Autodesk Inventor part; units mm, degrees
ref_plane "YZ Plane" through (0, 0, 0) normal (1, 0, 0) x (0, 1, 0)
ref_plane "XZ Plane" through (0, 0, 0) normal (0, 1, 0) x (-1, 0, 0)
ref_plane "XY Plane" through (0, 0, 0) normal (0, 0, 1) x (1, 0, 0)
sketch "スケッチ1" plane through (0, 0, 0) normal (0, 1, 0) x (-1, 0, 0)
  circle A0 centre (0, 0) radius 125
  dimension "d0" = 250
extrude "押し出し1" add sketch "スケッチ1" along normal blind 3
sketch "スケッチ2" plane through (0, 3, 0) normal (0, 1, 0) x (1, 0, 0)
  circle A0 centre (0, 0) radius 125
  circle A1 centre (0, 0) radius 117.5
  dimension "d3" = 250
  dimension "d4" = 235
extrude "押し出し2" add sketch "スケッチ2" along normal blind 144
sketch "スケッチ3" plane through (0, 147, 0) normal (0, 1, 0) x (1, 0, 0)
  circle A0 centre (0, 0) radius 125
extrude "押し出し3" add sketch "スケッチ3" along normal blind 3
sketch "スケッチ4" plane through (0, 150, 0) normal (0, 1, 0) x (1, 0, 0)
  circle A0 centre (60, 60) radius 15
  point P0 (0, 0)
  dimension "d9" = 30
  dimension "d10" = 60
  dimension "d11" = 60
extrude "押し出し4" cut sketch "スケッチ4" against normal through all
properties part number "dummy1"
Could you check a few things on this model? Use its own coordinates, in mm. A direction names the side the tool comes from. Round coordinates to 2 decimals unless told otherwise and drop trailing zeros. Order: outer loops, then holes, each group sorted by start corner. A loop starts at its lowest first (then second) coordinate and runs counter-clockwise, first axis right, second up. Notation, with made-up numbers: M 88,54.25 L 136,54.25 A11 cw 136,71.25 Z; hole C -38.75,34 d5. An arc over 180 degrees is marked long. One line per question, with ' | ' between items. Start each with the question number.
(1) For faces 1 (the face through (2, 3, 2)), 2 (the face through (-2, 150, -2)), which set-ups out of +Z, -Z, +X, -X, +Y, -Y let a thin tool reach every point of the face, with its end or its side?
(2) Suppose I cut it at B-B on y = 35.5. List the corners of the cut face in (x, z) for me, then the cut area to 3 significant figures.
(3) Please list where these lines run through material, in increasing order: line 1 along Y through (x, z) = (31.5, -79.5); line 2 along Z through (x, y) = (0, 70.5).
(4) Suppose I cut it at D-D on z = -12. List the corners of the cut face in (x, y) for me.
(5) Suppose I cut it at A-A on z = -38. List the corners of the cut face in (x, y) for me.
(6) Thinking about a two-plate mould opening in Z: for faces 3 (the face through (56.748, 1.521, -45.357)), 4 (the face through (-2, 147, -2)), 5 (the face through (2, 0, 2)), which applies, +Z half, -Z half, draft (parallel to the pull), parting line (faces both ways), or undercut?
(7) For P1, Ø5, axis at y = 130.5, z = 66.5, coming from the +X side; P2, Ø10, axis at y = 113, z = -94.5, coming from the -X side; P3, Ø1, axis at y = 16, z = -75, coming from the -X side; P4, Ø24, axis at x = 60, z = -60, coming from the -Y side, each with a flat end and sliding along its axis, tell me the tip position at first contact or that it passes through.
Geometry results:
1) face 1: none | face 2: +Z, -Z, +X, -X, +Y
2) outline: C 0,0 d250; hole C 0,0 d235 | area: 5,710 mm²
3) line 1: 0 to 3, 147 to 150 | line 2: -125 to -117.5, 117.5 to 125
4) outline: M -124.42,0 L 124.42,0 L 124.42,150 L -124.42,150 Z; hole M -116.89,3 L 116.89,3 L 116.89,147 L -116.89,147 Z
5) outline: M -119.08,0 L 119.08,0 L 119.08,150 L -119.08,150 Z; hole M -111.19,3 L 111.19,3 L 111.19,147 L -111.19,147 Z
6) face 3: undercut | face 4: undercut | face 5: draft
7) P1: x = 107.37 | P2: x = -87.26 | P3: x = -100.37 | P4: through
